from build123d import *

# Parameters (mm, degrees)
F1_DEPTH  = 1.778
F2_R      = 16.51
F3_DEPTH  = 1.27
F4_R      = 13.97
F5_DEPTH  = 1.778
F6_R      = 11.43
F7_DEPTH  = 1.27
F8_R      = 8.89
F9_DEPTH  = 1.778
F10_R     = 6.35
F11_DEPTH = 1.27
F12_R     = 3.81
F13_DEPTH = 1.524
F14_R     = 1.905
F15_DEPTH = 1.27
F16_R     = 0.635
F17_DEPTH = 0.889
F18_R     = 1.0795
F19_DEPTH = 1.778
F21_DEPTH = 1.27
F23_DEPTH = 1.778
F25_DEPTH = 1.27
F27_DEPTH = 1.778
F29_DEPTH = 1.27
F31_DEPTH = 1.778
F33_DEPTH = 1.27
F35_DEPTH = 0.889


with BuildPart() as f1:
    # F0 (on Right) → F1 (new body)
    with BuildSketch(Plane.YZ):
        with BuildLine():
            ThreePointArc((-19.05, 0), (-5.5796158184, 5.5796158184), (0, 19.05))
            ThreePointArc((0, 19.05), (-5.5796158184, 32.5203841816), (-19.05, 38.1))
            ThreePointArc((-19.05, 38.1), (-32.5203841816, 32.5203841816), (-38.1, 19.05))
            ThreePointArc((-38.1, 19.05), (-32.5203841816, 5.5796158184), (-19.05, 0))
        make_face()
    extrude(amount=F1_DEPTH)

    # F2 (on face) → F3 (join)
    with BuildSketch(Plane.YZ.offset(1.778)):
        with Locations((-19.05, 19.05)):
            Circle(F2_R)
    extrude(amount=F3_DEPTH)

    # F4 (on face) → F5 (join)
    with BuildSketch(Plane.YZ.offset(3.048)):
        with Locations((-19.05, 19.05)):
            Circle(F4_R)
    extrude(amount=F5_DEPTH)

    # F6 (on face) → F7 (join)
    with BuildSketch(Plane.YZ.offset(4.826)):
        with Locations((-19.05, 19.05)):
            Circle(F6_R)
    extrude(amount=F7_DEPTH)

    # F8 (on face) → F9 (join)
    with BuildSketch(Plane.YZ.offset(6.096)):
        with Locations((-19.05, 19.05)):
            Circle(F8_R)
    extrude(amount=F9_DEPTH)

    # F10 (on face) → F11 (join)
    with BuildSketch(Plane.YZ.offset(7.874)):
        with Locations((-19.05, 19.05)):
            Circle(F10_R)
    extrude(amount=F11_DEPTH)

    # F12 (on face) → F13 (join)
    with BuildSketch(Plane.YZ.offset(9.144)):
        with Locations((-19.05, 19.05)):
            Circle(F12_R)
    extrude(amount=F13_DEPTH)

    # F14 (on face) → F15 (join)
    with BuildSketch(Plane.YZ.offset(10.668)):
        with Locations((-19.05, 19.05)):
            Circle(F14_R)
    extrude(amount=F15_DEPTH)

    # F16 (on face) → F17 (join)
    with BuildSketch(Plane.YZ.offset(11.938)):
        with Locations((-19.05, 19.05)):
            Circle(F16_R)
    extrude(amount=F17_DEPTH)

    # F18 (on face) → F19 (cut)
    with BuildSketch(Plane.YZ.offset(1.778)):
        with Locations((-35.6285501971, 25.4737715009)):
            Circle(F18_R)
    extrude(amount=-F19_DEPTH, mode=Mode.SUBTRACT)

    # F20 (on face) → F21 (join)
    with BuildSketch(Plane(origin=(0, 0, 0), x_dir=(0, -1, 0), z_dir=(-1, 0, 0))):
        with BuildLine():
            ThreePointArc((19.05, 35.56), (2.54, 19.05), (19.05, 2.54))
            Line((19.05, 2.54), (19.05, 35.56))
        make_face()
        with BuildLine():
            Line((19.05, 35.56), (19.05, 2.54))
            ThreePointArc((19.05, 2.54), (30.7243329574, 7.3756670426), (35.56, 19.05))
            ThreePointArc((35.56, 19.05), (30.7243329574, 30.7243329574), (19.05, 35.56))
        make_face()
    extrude(amount=F21_DEPTH)

    # F22 (on face) → F23 (join)
    with BuildSketch(Plane(origin=(-1.27, 0, 0), x_dir=(0, -1, 0), z_dir=(-1, 0, 0))):
        with BuildLine():
            ThreePointArc((19.05, 33.02), (5.08, 19.05), (19.05, 5.08))
            Line((19.05, 5.08), (19.05, 33.02))
        make_face()
        with BuildLine():
            Line((19.05, 33.02), (19.05, 5.08))
            ThreePointArc((19.05, 5.08), (28.9282817332, 9.1717182668), (33.02, 19.05))
            ThreePointArc((33.02, 19.05), (28.9282817332, 28.9282817332), (19.05, 33.02))
        make_face()
    extrude(amount=F23_DEPTH)

    # F24 (on face) → F25 (join)
    with BuildSketch(Plane(origin=(-3.048, 0, 0), x_dir=(0, -1, 0), z_dir=(-1, 0, 0))):
        with BuildLine():
            Line((19.05, 30.48), (19.05, 7.62))
            ThreePointArc((19.05, 7.62), (27.132230509, 10.967769491), (30.48, 19.05))
            ThreePointArc((30.48, 19.05), (27.132230509, 27.132230509), (19.05, 30.48))
        make_face()
        with BuildLine():
            ThreePointArc((19.05, 30.48), (7.62, 19.05), (19.05, 7.62))
            Line((19.05, 7.62), (19.05, 30.48))
        make_face()
    extrude(amount=F25_DEPTH)

    # F26 (on face) → F27 (join)
    with BuildSketch(Plane(origin=(-4.318, 0, 0), x_dir=(0, -1, 0), z_dir=(-1, 0, 0))):
        with BuildLine():
            ThreePointArc((19.05, 27.94), (10.16, 19.05), (19.05, 10.16))
            Line((19.05, 10.16), (19.05, 27.94))
        make_face()
        with BuildLine():
            Line((19.05, 27.94), (19.05, 10.16))
            ThreePointArc((19.05, 10.16), (25.3361792847, 12.7638207153), (27.94, 19.05))
            ThreePointArc((27.94, 19.05), (25.3361792847, 25.3361792847), (19.05, 27.94))
        make_face()
    extrude(amount=F27_DEPTH)

    # F28 (on face) → F29 (join)
    with BuildSketch(Plane(origin=(-6.096, 0, 0), x_dir=(0, -1, 0), z_dir=(-1, 0, 0))):
        with BuildLine():
            ThreePointArc((19.05, 25.4), (12.7, 19.05), (19.05, 12.7))
            Line((19.05, 12.7), (19.05, 25.4))
        make_face()
        with BuildLine():
            Line((19.05, 25.4), (19.05, 12.7))
            ThreePointArc((19.05, 12.7), (23.5401280605, 14.5598719395), (25.4, 19.05))
            ThreePointArc((25.4, 19.05), (23.5401280605, 23.5401280605), (19.05, 25.4))
        make_face()
    extrude(amount=F29_DEPTH)

    # F30 (on face) → F31 (join)
    with BuildSketch(Plane(origin=(-7.366, 0, 0), x_dir=(0, -1, 0), z_dir=(-1, 0, 0))):
        with BuildLine():
            ThreePointArc((19.05, 22.86), (15.24, 19.05), (19.05, 15.24))
            Line((19.05, 15.24), (19.05, 22.86))
        make_face()
        with BuildLine():
            Line((19.05, 22.86), (19.05, 15.24))
            ThreePointArc((19.05, 15.24), (21.7440768363, 16.3559231637), (22.86, 19.05))
            ThreePointArc((22.86, 19.05), (21.7440768363, 21.7440768363), (19.05, 22.86))
        make_face()
    extrude(amount=F31_DEPTH)

    # F32 (on face) → F33 (join)
    with BuildSketch(Plane(origin=(-9.144, 0, 0), x_dir=(0, -1, 0), z_dir=(-1, 0, 0))):
        with BuildLine():
            Line((19.05, 20.955), (19.05, 17.145))
            ThreePointArc((19.05, 17.145), (20.3970384182, 17.7029615818), (20.955, 19.05))
            ThreePointArc((20.955, 19.05), (20.3970384182, 20.3970384182), (19.05, 20.955))
        make_face()
        with BuildLine():
            ThreePointArc((19.05, 20.955), (17.145, 19.05), (19.05, 17.145))
            Line((19.05, 17.145), (19.05, 20.955))
        make_face()
    extrude(amount=F33_DEPTH)

    # F34 (on face) → F35 (join)
    with BuildSketch(Plane(origin=(-10.414, 0, 0), x_dir=(0, -1, 0), z_dir=(-1, 0, 0))):
        with BuildLine():
            Line((19.05, 19.685), (19.05, 18.415))
            ThreePointArc((19.05, 18.415), (19.4990128061, 18.6009871939), (19.685, 19.05))
            ThreePointArc((19.685, 19.05), (19.4990128061, 19.4990128061), (19.05, 19.685))
        make_face()
        with BuildLine():
            ThreePointArc((19.05, 19.685), (18.415, 19.05), (19.05, 18.415))
            Line((19.05, 18.415), (19.05, 19.685))
        make_face()
    extrude(amount=F35_DEPTH)


solid = f1.part
Geometry: final body of the model. Coordinates: model frame, mm. A direction names the side the tool comes from. Give positions to 0.01 mm unless a question says otherwise; leave off trailing zeros. Write each loop counter-clockwise with the first axis right and the second up, starting at its lowest first coordinate (ties: lowest second). Pieces come first, ordered by that corner, then holes. Notation, with made-up numbers: M 60,61 L 78,61 A28 cw 78,98 Z; hole C -17.75,43.5 d10. An arc over 180 degrees is marked long. Answer in a Markdown table with one row per item. Add a question column.
(1) Section A-A on z = 30. Return loops of the section in (x, y), and give its area (3 significant figures).
(2) First-contact query: pin 1 (12 mm diameter, centred on x = 8.5, y = -6, fed in from -Z); pin 2 (2 mm diameter, centred on y = -21, z = 32.5, fed in from +X); pin 3 (6 mm diameter, centred on x = 2, y = -23.5, fed in from -Z). Flat tips, straight axial feed; report the tip coordinate or a pass-through.
(3) Section C-C on y = -29.5. Return loops of the section in (x, z), and give its area (3 significant figures).
(4) Ray query, line 1 (X direction, y = -19.5, z = 15); line 2 (X direction, y = -6, z = 7); line 3 (Z direction, x = -2.25, y = -18.5). Return the intervals inside material, ascending.
(5) Reachability of faces 1 (the flat face through (-1.27, -23, 33)), 2 (the flat face through (12.827, -19, 19)), 3 (the flat face through (9.144, -16, 16)) from +Z, -Z, +X, -X, +Y, -Y: full face, straight path, thin tool, end or side. Return the list, or none.
(6) Section D-D on x = 11.25. Return loops of the section in (y, z) (3 decimals), and give its area (3 significant figures).
(7) Section B-B on x = -6.75. Return loops of the section in (y, z), and give its area (3 significant figures).
Result set:
| question | item | result |
|---|---|---|
| 1 | outline | M -4.32,-22.33 L -3.05,-22.33 L -3.05,-27.73 L -1.27,-27.73 L -1.27,-31.41 L 0,-31.41 L 0,-34.64 L 1.78,-34.64 L 1.78,-31.41 L 3.05,-31.41 L 3.05,-27.73 L 4.83,-27.73 L 4.83,-22.33 L 6.1,-22.33 L 6.1,-15.77 L 4.83,-15.77 L 4.83,-10.37 L 3.05,-10.37 L 3.05,-6.69 L 1.78,-6.69 L 1.78,-3.46 L 0,-3.46 L 0,-6.69 L -1.27,-6.69 L -1.27,-10.37 L -3.05,-10.37 L -3.05,-15.77 L -4.32,-15.77 Z |
| 1 | area | 197 mm^2 |
| 2 | pin 1 | stops at z = 6.35 |
| 2 | pin 2 | stops at x = 4.83 |
| 2 | pin 3 | stops at z = 0.06 |
| 3 | outline | M -4.32,14.42 L -3.05,14.42 L -3.05,9.78 L -1.27,9.78 L -1.27,6.27 L 0,6.27 L 0,3.12 L 1.78,3.12 L 1.78,6.27 L 3.05,6.27 L 3.05,9.78 L 4.83,9.78 L 4.83,14.42 L 6.1,14.42 L 6.1,23.68 L 4.83,23.68 L 4.83,28.32 L 3.05,28.32 L 3.05,31.83 L 1.78,31.83 L 1.78,34.98 L 0,34.98 L 0,31.83 L -1.27,31.83 L -1.27,28.32 L -3.05,28.32 L -3.05,23.68 L -4.32,23.68 Z |
| 3 | area | 211 mm^2 |
| 4 | line 1 | x = -7.37 to 9.14 |
| 4 | line 2 | x = 0 to 1.78 |
| 4 | line 3 | z = 5.09 to 33.01 |
| 5 | face 1 | -X |
| 5 | face 2 | +Z, -Z, +X, +Y, -Y |
| 5 | face 3 | +X |
| 6 | outline | C -19.05,19.05 d3.81 |
| 6 | area | 11.4 mm^2 |
| 7 | outline | C -19.05,19.05 d12.7 |
| 7 | area | 127 mm^2 |
